Geometry: see drawing. Coordinates: mm, zero at the bounding-box minimum. A direction names the side the tool comes from. Give positions to 0.01 mm unless a question says otherwise; leave off trailing zeros. Order: outer loops, then holes, each group sorted by start corner. A loop starts at its lowest first (then second) coordinate and runs counter-clockwise, first axis right, second up. Notation, with made-up numbers: (-27.5, 52) - (19.5, 52) arc R17 cw to (19.5, 73) - close; hole circle Ø1 at (-32, 37.25). An arc over 180 degrees is marked (long way). Write item = value, one per line. Start each with the question number.
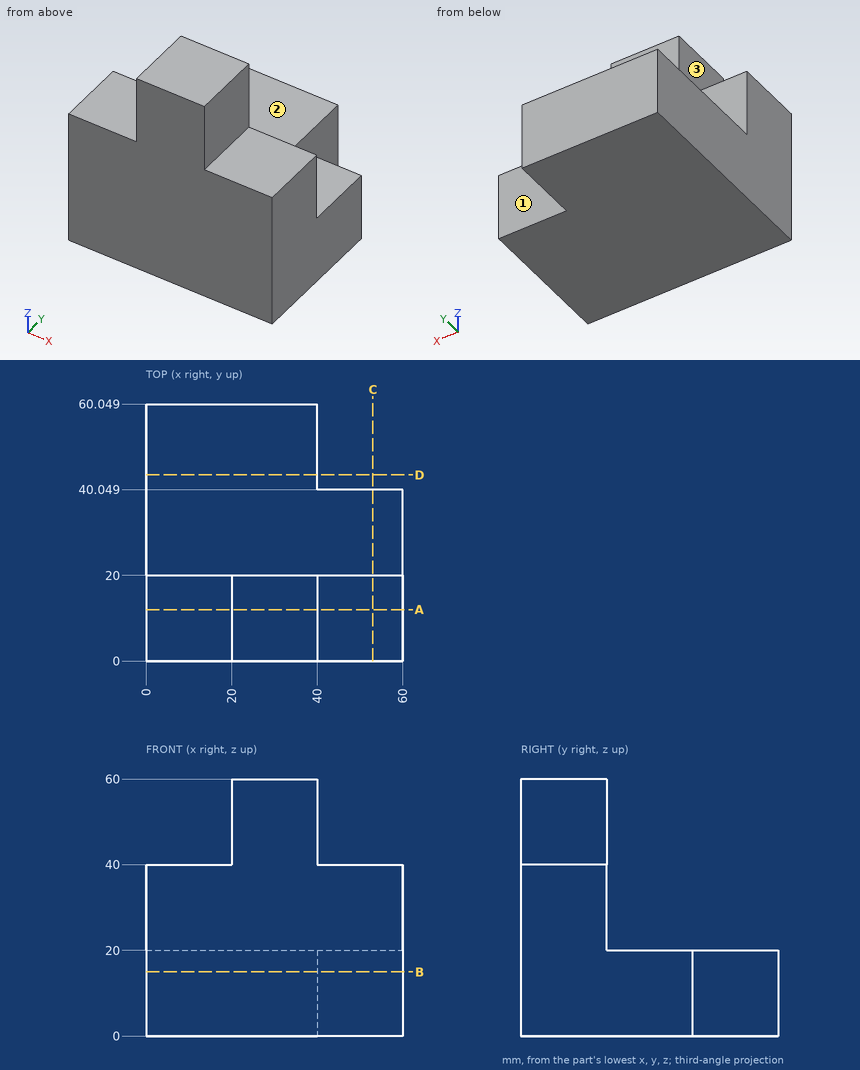
Q1. Section D-D, the plane y = 43.5. Return the cut outline in (x, z), then the cut area to 3 significant figures.
Q2. Section B-B, the plane z = 15. Return the cut outline in (x, y), then the cut area to 3 significant figures.
Q3. Set-up query: the marked faces 1, 2 and 3. Return all of +Z, -Z, +X, -X, +Y, -Y with unobstructed straight access to the full face (end or side cutting, diameter ignored); none if empty.
Q4. Section A-A, the plane y = 12. Return the cut outline in (x, z), then the cut area to 3 significant figures.
Q5. Section C-C, the plane x = 53. Return the cut outline in (y, z), then the cut area to 3 significant figures.
Q6. Contact query for flat-ended pins moving along their axis: pin 1 (20 mm diameter, centred on x = 25, y = 41.5, fed in from +Z); pin 2 (4 mm diameter, centred on y = 21.5, z = 43.5, fed in from +X); pin 3 (2 mm diameter, centred on x = 18, z = 46.5, fed in from +Y); pin 4 (12 mm diameter, centred on x = 35, z = 37, fed in from +Y). Output: stop coordinate, or through.
Q7. Material intervals for line 1 along Y through (x, z) = (34, 22.5); line 2 along Y through (x, z) = (47, 15.5); line 3 along Z through (x, y) = (6, 16), sorted ascending. Write a range as from..to.
The answers:
q1.outline = (0, 0) - (40, 0) - (40, 20) - (0, 20) - close
q1.area = 800 mm²
q2.outline = (0, 0) - (60, 0) - (60, 40.05) - (40, 40.05) - (40, 60.05) - (0, 60.05) - close
q2.area = 3,200 mm²
q3.face_1 = +Z, -Z, +X, +Y
q3.face_2 = +Z, +X, -X, +Y
q3.face_3 = +Z, -X, +Y, -Y
q4.outline = (0, 0) - (60, 0) - (60, 40) - (40, 40) - (40, 60) - (20, 60) - (20, 40) - (0, 40) - close
q4.area = 2,800 mm²
q5.outline = (0, 0) - (40.05, 0) - (40.05, 20) - (20, 20) - (20, 40) - (0, 40) - close
q5.area = 1,200 mm²
q6.pin_1 = 20
q6.pin_2 = 40
q6.pin_3 = through
q6.pin_4 = 20
q7.line_1 = 0..20
q7.line_2 = 0..40.05
q7.line_3 = 0..40
